```python
from build123d import *

# Parameters (mm, degrees)
SKETCH_1_W      = 494
SKETCH_1_H      = 10
SKETCH_2_R      = 10
EXTRUDE_1_DEPTH = 76


with BuildPart() as part:
    # 草图1 → 旋转1 (revolve)
    with BuildSketch(Plane.XY):
        Polygon((-265, 0), (-265, 10), (-253, 10), (-253, 12), (-250, 12), (-250, 25), (250, 25), (250, 12), (253, 12), (253, 10), (303, 10), (303, 0), align=None)
        with Locations((0, 17)):
            Rectangle(SKETCH_1_W, SKETCH_1_H, mode=Mode.SUBTRACT)
    revolve(axis=Axis((303, 0, 0), (-1, 0, 0)))

    # 草图2 → 凸台-拉伸1 (add)
    with BuildSketch(Plane.ZY.offset(265)):
        with Locations(Location((0, 0, 0), (0, 0, 90))):
            Circle(SKETCH_2_R)
    extrude(amount=EXTRUDE_1_DEPTH)


solid = part.part
```
Can you work these out from the model? Positions are in its coordinate system, mm. A direction names the side the tool comes from. Round coordinates to 2 decimals unless told otherwise and drop trailing zeros. Order: outer loops, then holes, each group sorted by start corner. A loop starts at its lowest first (then second) coordinate and runs counter-clockwise, first axis right, second up. Notation, with made-up numbers: (24, -1.5) -> (59, -1.5) arc R27 cw to (59, 15.5) -> close; hole circle Ø5 at (64, 22). An arc over 180 degrees is marked (long way). Return JSON: item names as keys, results as strings. Group by question number.
1. Will these pins go through, and if not, where does the flat tip stop? pin 1 (12 mm diameter, centred on x = -117, z = -4, fed in from +Y); pin 2 (4 mm diameter, centred on y = -9.5, z = -12, fed in from -X); pin 3 (5 mm diameter, centred on y = -7, z = 17.5, fed in from +X); pin 4 (3 mm diameter, centred on x = 60.5, z = -5.5, fed in from -Y).
2. If we section it at A-A, the plane x = 95.5: Write out the boundary of the cut face in (y, z).
3. We'd pull the mould along Z, two halves only. Please class faces 1 (the face through (251.52, -11.99, -0.53)), 2 (the face through (3.458, -4.769, 21.477)), 3 (the face through (250, -6, 11)): released by +Z, released by -Z, zero draft, split by the parting line, or undercut.
4. Which directions (+Z, -Z, +X, -X, +Y, -Y) give clear straight access to the entire face, cutting with the end or side of a thin tool? Please do faces 4 (the face through (-251.48, -11.99, -0.53)), 5 (the face through (253, -5, -9)), 6 (the face through (247, -9, 9)).
5. I need wall thicknesses on line 1 (Z direction, x = -104, y = 0); line 2 (Y direction, x = -141, z = -3). Which ranges of each line are inside material? Lowest first, please. Write a range as [from, to].
6. If we section it at B-B, the plane y = 0: Write out the boundary of the cut face in (x, z).
Output values:
{
 "1": {"pin 1": "y = 25", "pin 2": "x = -250", "pin 3": "x = 250", "pin 4": "y = -24.68"},
 "2": {"outline": "circle Ø50 at (0, 0); circle Ø24 at (0, 0); hole circle Ø44 at (0, 0)"},
 "3": {"face 1": "split by the parting line", "face 2": "undercut", "face 3": "zero draft"},
 "4": {"face 4": "-X", "face 5": "+X", "face 6": "none"},
 "5": {"line 1": "[-25, -22], [-12, 12], [22, 25]", "line 2": "[-24.82, -21.79], [-11.62, 11.62], [21.79, 24.82]"},
 "6": {"outline": "(-341, -10) -> (-253, -10) -> (-253, -12) -> (-250, -12) -> (-250, -25) -> (250, -25) -> (250, -12) -> (253, -12) -> (253, -10) -> (303, -10) -> (303, 10) -> (253, 10) -> (253, 12) -> (250, 12) -> (250, 25) -> (-250, 25) -> (-250, 12) -> (-253, 12) -> (-253, 10) -> (-341, 10) -> close; hole (-247, -22) -> (247, -22) -> (247, -12) -> (-247, -12) -> close; hole (-247, 12) -> (247, 12) -> (247, 22) -> (-247, 22) -> close"}
}
